from build123d import *

# Parameters (mm, degrees)
F0_R     = 4.064
F1_DEPTH = 152.4
F2_R     = 6.35
F2_R_2   = 4.064
F3_DEPTH = 7.62
F4_R     = 6.35
F4_R_2   = 4.064
F5_DEPTH = 7.62
F6_SIZE  = 2.28599


# Not quite as in the source:
# - a fillet or chamfer is up to 0.001 mm smaller than in the source, because OpenCascade refuses the exact size


with BuildPart() as f1:
    # F0 (on Top) → F1 (new body)
    with BuildSketch(Plane.XY):
        Circle(F0_R)
    extrude(amount=F1_DEPTH)

    # F2 (on face) → F3 (join)
    with BuildSketch(Plane.XY.offset(152.4)):
        Circle(F2_R)
        Circle(F2_R_2, mode=Mode.SUBTRACT)
        Circle(F2_R_2)
    extrude(amount=F3_DEPTH)

    # F4 (on face) → F5 (join)
    with BuildSketch(Plane(origin=(0, 0, 0), x_dir=(1, 0, 0), z_dir=(0, 0, -1))):
        Circle(F4_R)
        Circle(F4_R_2, mode=Mode.SUBTRACT)
        Circle(F4_R_2)
    extrude(amount=F5_DEPTH)

    # F6 (size 2.286 in the source; OpenCascade refuses exactly that, so slightly less here)
    f6_edges = [f1.edges().sort_by_distance(p)[0] for p in [
        (-6.35, 0, 0),
        (-6.35, 0, 152.4),
    ]]
    chamfer(f6_edges, length=F6_SIZE)


solid = f1.part
The model under review builds one solid part; all positions refer to its coordinate system, in mm. A direction names the side the tool comes from. Give positions to 0.01 mm unless a question says otherwise; leave off trailing zeros. Order: outer loops, then holes, each group sorted by start corner. A loop starts at its lowest first (then second) coordinate and runs counter-clockwise, first axis right, second up. Notation, with made-up numbers: M 8,-24 L 49,-24 A21 cw 49,-6 Z; hole C -21.75,71.25 d8. An arc over 180 degrees is marked long. Use one line per item in the form item = value. Start each with the question number.
Item 1: Insertion check: pin 1 Ø1.5 at (y, z) = (-1.5, 23.5) entering from +X; pin 2 Ø1.5 at (x, z) = (0, 83.5) entering from +Y; pin 3 Ø4 at (x, z) = (3, 65) entering from -Y. Each pin has a flat end and moves straight along its axis. Give the tip position at first contact, or say it passes through.
Item 2: To check wall thickness, follow line 1 along Z through (x, y) = (-1.25, -4); line 2 along Z through (x, y) = (-2.75, -4.5); line 3 along Y through (x, z) = (-0.5, 89). State the ranges of each line that lie inside material, in increasing order. Write a range as from..to.
Item 3: For faces 1 (the cylindrical face through (-1.38, 6.2, -4.92)), 2 (the conical face through (-3.31, 2.54, -0.11)), list the 3-axis set-ups (+Z, -Z, +X, -X, +Y, -Y) from which the entire face can be reached by the end or side of a thin tool; tool diameter is ignored.
Item 4: We need section C-C on z = 109. Give the boundary of the cut face in (x, y).
Completed:
q1.pin_1 = 3.99
q1.pin_2 = 4.06
q1.pin_3 = -3.94
q2.line_1 = -7.62..-0.13, 152.53..160.02
q2.line_2 = -7.62..-1.21, 153.61..160.02
q2.line_3 = -4.03..4.03
q3.face_1 = +Z, -Z
q3.face_2 = none
q4.outline = C 0,0 d8.13
